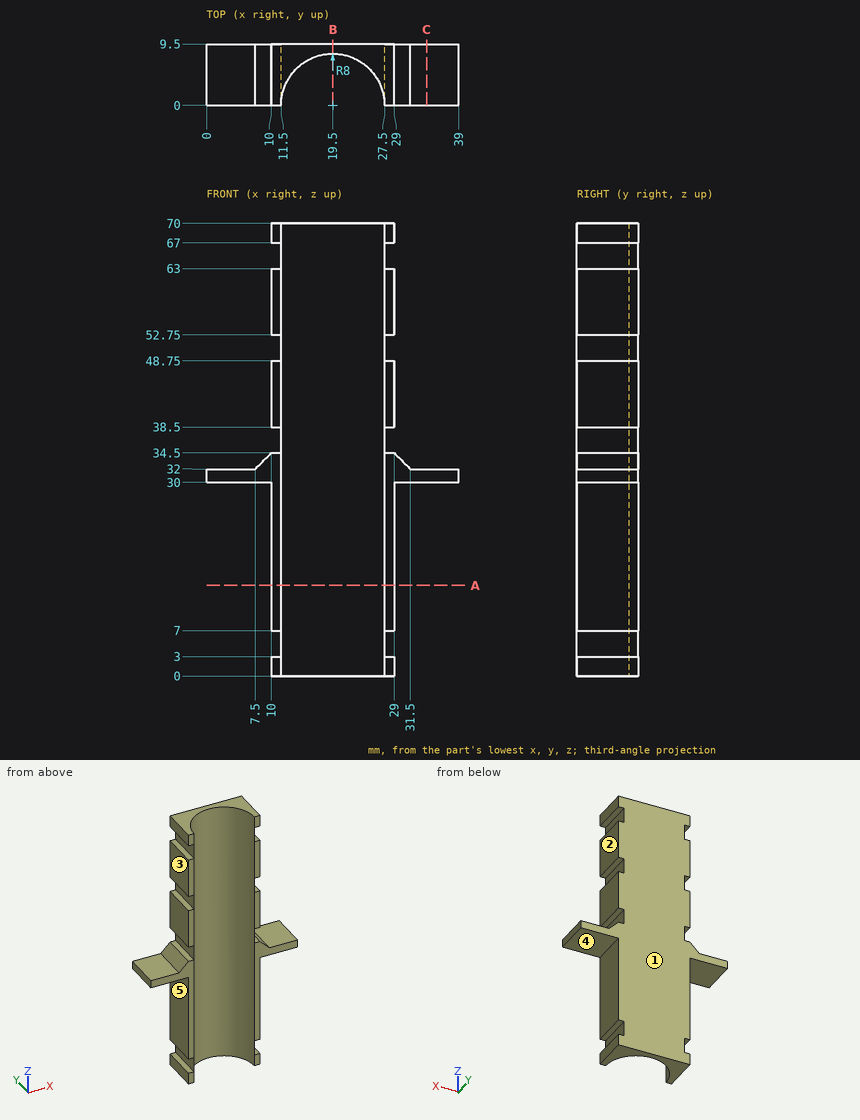
Answer from the drawing. Dimensions are ordinates in mm from the lowest x, y and z of the part. A direction names the side the tool comes from. Coordinates: 2 decimals unless noted, no trailing zeros. Loops run counter-clockwise (first coordinate to the right, second up) from the corner with the lowest first, then second, coordinate; pieces in that order, holes last. Notation, with made-up numbers: (41, 13) - (76, 13) arc R28 cw to (76, 50) - close; hole circle Ø1 at (29.5, 16). An arc over 180 degrees is marked (long way). Use a Markdown table: item, result.
Item 1: Find section C-C, the plane x = 34. Determine the outline of the cut face in (y, z), and give its area (3 significant figures).
Evaluation:
| item | result |
|---|---|
| outline | (0, 30) - (9.5, 30) - (9.5, 32) - (0, 32) - close |
| area | 19.0 mm2 |
Item 2: For the marked faces 1, 2, 3, 4 and 5, determine the directions among +Z, -Z, +X, -X, +Y, -Y from which every point of the face is accessible in a straight line to the end or side of a thin tool.
Evaluation:
| item | result |
|---|---|
| face 1 | +Z, -Z, +X, -X, +Y |
| face 2 | +Z, +X, +Y, -Y |
| face 3 | +Z, -X, +Y, -Y |
| face 4 | -Z, +X, +Y, -Y |
| face 5 | -Z, -X, +Y, -Y |
Item 3: Find section B-B, the plane x = 19.5. Determine the outline of the cut face in (y, z).
Evaluation:
| item | result |
|---|---|
| outline | (8, 0) - (9.5, 0) - (9.5, 70) - (8, 70) - close |
Item 4: Find section A-A, the plane z = 14. Determine the outline of the cut face in (x, y), and give its area (3 significant figures).
Evaluation:
| item | result |
|---|---|
| outline | (10, 0) - (11.5, 0) arc R8 cw to (27.5, 0) - (29, 0) - (29, 9.5) - (10, 9.5) - close |
| area | 80.0 mm2 |
Item 5: Given pin 1 Ø3 at (y, z) = (2.5, 39) entering from -X; pin 2 Ø2 at (y, z) = (4, 60.5) entering from +X; pin 3 Ø8 at (x, z) = (5, 11.5) entering from +Y; pin 4 Ø4 at (x, y) = (5.5, 4) entering from -Z, each flat-ended and moving along its own axis, determine where each tip first touches the part or whether it passes through.
Evaluation:
| item | result |
|---|---|
| pin 1 | stops at x = 10 |
| pin 2 | stops at x = 29 |
| pin 3 | passes through |
| pin 4 | stops at z = 30 |
Item 6: Consider probe 1 along Z at (x, y) = (28, 1); probe 2 along Z at (x, y) = (3.5, 0.5); probe 3 along X at (y, z) = (5.25, 59). Determine where each line is inside the solid, lowest interval first. Write a range as from..to.
Evaluation:
| item | result |
|---|---|
| probe 1 | z = 0..3, 7..34.5, 38.5..48.75, 52.75..63, 67..70 |
| probe 2 | z = 30..32 |
| probe 3 | x = 10..13.46, 25.54..29 |
